from build123d import *

# Parameters (mm, degrees)
SCHIZZO1_R                   = 0.61
SCHIZZO1_R_2                 = 0.985
ESTRUSIONE_ESTRUSIONE1_DEPTH = 1.74
ESTRUSIONE_ESTRUSIONE2_START = -1.74
SCHIZZO2_R                   = 3.51
ESTRUSIONE_ESTRUSIONE2_DEPTH = 4.38
ESTRUSIONE_ESTRUSIONE3_START = -4.38
SCHIZZO3_R                   = 2.7
ESTRUSIONE_ESTRUSIONE3_DEPTH = 5.05
SCHIZZO4_R                   = 2.45
TAGLIO_ESTRUSIONE1_DEPTH     = 2.33
SCHIZZO5_R                   = 2
TAGLIO_ESTRUSIONE2_DEPTH     = 1.35
TAGLIO_ESTRUSIONE3_REACH     = 17.929
SCHIZZO6_R                   = 1.06


with BuildPart() as part:
    # Schizzo1 → Estrusione-Estrusione1 (new body)
    with BuildSketch(Plane.XY):
        with BuildLine():
            Line((12.790555997, 2.491942474), (0.28158062, 3.498687233))
            ThreePointArc((0.28158062, 3.498687233), (-3.51, 0), (0.28158062, -3.498687233))
            Line((0.28158062, -3.498687233), (12.790555997, -2.491942474))
            ThreePointArc((12.790555997, -2.491942474), (15.09, 0), (12.790555997, 2.491942474))
        make_face()
        with Locations((9.49, 0)):
            Circle(SCHIZZO1_R, mode=Mode.SUBTRACT)
        with Locations((6.19, 0)):
            Circle(SCHIZZO1_R, mode=Mode.SUBTRACT)
        with Locations((12.59, 0)):
            Circle(SCHIZZO1_R_2, mode=Mode.SUBTRACT)
    extrude(amount=ESTRUSIONE_ESTRUSIONE1_DEPTH)

    # Schizzo2 → Estrusione-Estrusione2 (add)
    with BuildSketch(Plane.XY.offset(1.74).offset(ESTRUSIONE_ESTRUSIONE2_START)):
        with Locations(Location((0, 0, 0), (0, 0, 274.601349332))):
            Circle(SCHIZZO2_R)
    extrude(amount=ESTRUSIONE_ESTRUSIONE2_DEPTH)

    # Schizzo3 → Estrusione-Estrusione3 (add)
    with BuildSketch(Plane(origin=(0, 0, 0), x_dir=(-1, 0, 0), z_dir=(0, 0, -1)).offset(ESTRUSIONE_ESTRUSIONE3_START)):
        with Locations(Location((0, 0, 0), (0, 0, 180))):
            Circle(SCHIZZO3_R)
    extrude(amount=ESTRUSIONE_ESTRUSIONE3_DEPTH)

    # Schizzo4 → Taglio-Estrusione1 (cut)
    with BuildSketch(Plane.XY.offset(4.38)):
        Circle(SCHIZZO4_R)
    extrude(amount=-TAGLIO_ESTRUSIONE1_DEPTH, mode=Mode.SUBTRACT)

    # Schizzo5 → Taglio-Estrusione2 (cut)
    with BuildSketch(Plane(origin=(0, 0, -0.67), x_dir=(-1, 0, 0), z_dir=(0, 0, -1))):
        Circle(SCHIZZO5_R)
    extrude(amount=-TAGLIO_ESTRUSIONE2_DEPTH, mode=Mode.SUBTRACT)

    # Schizzo6 → Taglio-Estrusione3 (cut, up to next)
    with BuildSketch(Plane(origin=(0, 0, 0.68), x_dir=(-1, 0, 0), z_dir=(0, 0, -1)), mode=Mode.PRIVATE) as taglio_estrusione3_sk1:
        Circle(SCHIZZO6_R)
    taglio_estrusione3_tool1 = extrude(taglio_estrusione3_sk1.sketch, amount=-TAGLIO_ESTRUSIONE3_REACH, mode=Mode.PRIVATE) & part.part
    add(taglio_estrusione3_tool1.solids().sort_by_distance((0, 0, 0.68))[0], mode=Mode.SUBTRACT)


solid = part.part
Verification items for the finished model (mm, model axes). A direction names the side the tool comes from. Give positions to 0.01 mm unless a question says otherwise; leave off trailing zeros. Write each loop counter-clockwise with the first axis right and the second up, starting at its lowest first coordinate (ties: lowest second). Pieces come first, ordered by that corner, then holes.
(1) Cross-section at A-A (y = 0). State how many separate pieces and enclosed holes the cut face has, plus the area to 3 significant figures.
(2) Cross-section at B-B (x = 0). Enter the section's corners in (y, z).
(3) Material ranges on line 1 (Y direction, x = 0, z = 0.35); line 2 (Y direction, x = 0, z = 3.75); line 3 (Z direction, x = 5.5, y = 0.5), recorded low to high.
(4) Cross-section at D-D (x = 6.19). Enter the section's corners in (y, z).
(5) Mould release check, pull along Y, two halves, no side actions. Record for faces 1 (the face through (2, 2, 4.38)), 2 (the face through (6.62, 2.99, 0.86)), 3 (the face through (-0.5, -2.4, 3.2)): +Y half, -Y half, draft (parallel to the pull), parting line (faces both ways), or undercut.
(6) Access from +Z, -Z, +X, -X, +Y, -Y to the whole of each face (thin tool, end or side, straight path). Record for faces 4 (the face through (-3.477, 0.484, 2.646)), 5 (the face through (-2.143, 1.643, -0.33)), 6 (the face through (6.449, -3.002, 0.858)).
(7) Cross-section at C-C (z = 3.8). Enter the section's corners in (x, y).
(8) Gauge pin test, flat ends, axial feed: pin 1 (1.4 mm diameter, centred on x = 9.49, y = 0, fed in from +Z); pin 2 (1 mm diameter, centred on x = 0.5, z = 3, fed in from -Y); pin 3 (1.2 mm diameter, centred on x = 0, y = 1, fed in from -Z); pin 4 (3 mm diameter, centred on x = 5.5, z = 3, fed in from -Y). Record the tip position at first contact, or that the pin passes through.
Worked out:
1. separate pieces: 5
1. enclosed holes: 0
1. area: 27.1 mm2
2. outline: (-3.51, 0) - (-2.7, 0) - (-2.7, -0.67) - (-2, -0.67) - (-2, 0.68) - (-1.06, 0.68) - (-1.06, 2.05) - (-2.45, 2.05) - (-2.45, 4.38) - (-3.51, 4.38) - close; (1.06, 0.68) - (2, 0.68) - (2, -0.67) - (2.7, -0.67) - (2.7, 0) - (3.51, 0) - (3.51, 4.38) - (2.45, 4.38) - (2.45, 2.05) - (1.06, 2.05) - close
3. line 1: y = -3.51 to -2, 2 to 3.51
3. line 2: y = -3.51 to -2.45, 2.45 to 3.51
3. line 3: z = 0 to 1.74
4. outline: (-3.02, 0) - (-0.61, 0) - (-0.61, 1.74) - (-3.02, 1.74) - close; (0.61, 0) - (3.02, 0) - (3.02, 1.74) - (0.61, 1.74) - close
5. face 1: draft
5. face 2: +Y half
5. face 3: undercut
6. face 4: +Z
6. face 5: -Z
6. face 6: +Z, -Z, +X, -Y
7. outline: circle Ø7.02 at (0, 0); hole circle Ø4.9 at (0, 0)
8. pin 1: stops at z = 1.74
8. pin 2: stops at y = -3.51
8. pin 3: stops at z = 0.68
8. pin 4: stops at y = -3.14
